from build123d import *

# Parameters (mm, degrees)
SKETCH1_R           = 7.67
BOSS_EXTRUDE1_DEPTH = 127
FILLET1_R           = 10
SKETCH2_W           = 50.8
SKETCH2_H           = 70.745219222
CUT_EXTRUDE1_DEPTH  = 186.59628229


with BuildPart() as part:
    # Sketch1 → Boss-Extrude1 (new body)
    with BuildSketch(Plane.XY):
        with BuildLine():
            Line((-19.5, 76.2), (-19.5, 0))
            ThreePointArc((-19.5, 0), (-13.788582233, -13.788582233), (0, -19.5))
            Line((0, -19.5), (76.2, -19.5))
            ThreePointArc((76.2, -19.5), (95.7, 0), (76.2, 19.5))
            Line((76.2, 19.5), (19.5, 19.5))
            Line((19.5, 19.5), (19.5, 76.2))
            ThreePointArc((19.5, 76.2), (0, 95.7), (-19.5, 76.2))
        make_face()
        Circle(SKETCH1_R, mode=Mode.SUBTRACT)
        with Locations((0, 76.2)):
            Circle(SKETCH1_R, mode=Mode.SUBTRACT)
        with Locations((76.2, 0)):
            Circle(SKETCH1_R, mode=Mode.SUBTRACT)
    extrude(amount=BOSS_EXTRUDE1_DEPTH)

    # Fillet1
    fillet1_edges = [part.edges().sort_by_distance(p)[0] for p in [
        (19.5, 19.5, 63.5),
    ]]
    fillet(fillet1_edges, radius=FILLET1_R)

    # Sketch2 → Cut-Extrude1 (cut, symmetric)
    with BuildSketch(Plane(origin=(0, 0, 0), x_dir=(0, 0, -1), z_dir=(1, 0, 0))):
        with Locations((-63.5, 80.272609611)):
            Rectangle(SKETCH2_W, SKETCH2_H)
    cut_extrude1 = extrude(amount=CUT_EXTRUDE1_DEPTH, both=True, mode=Mode.SUBTRACT)

    # Mirror1: Cut-Extrude1 across plane
    add(cut_extrude1.mirror(Plane(origin=(0, 0, 0), x_dir=(0, 0, 1), z_dir=(-0.7071067811865512, 0.7071067811865438, 0))), mode=Mode.SUBTRACT)


solid = part.part
Source: CAD feature listing. Evaluate the final solid. Frame: model axes, mm. A direction names the side the tool comes from. Coordinates: 2 decimals unless noted, no trailing zeros. Order: outer loops, then holes, each group sorted by start corner. A loop starts at its lowest first (then second) coordinate and runs counter-clockwise, first axis right, second up. Notation, with made-up numbers: M -37.75,-18 L 4.25,-18 A17 ccw 4.25,-6 Z; hole C 9.5,-7 d5. An arc over 180 degrees is marked long. Write each question's results on one line, items separated by ' | '. Start each with the question number.
Item 1: Line query: probe 1 along Y at (x, z) = (0, 24); probe 2 along Z at (x, y) = (16, 60); probe 3 along Y at (x, z) = (76.2, 117). Output: solid intervals per line, ascending.
Item 2: Cut plane D-D (y = 72). Return loops of the section in (x, z).
Item 3: Draft query along X for faces 1 (the face through (-13.939, -13.636, 62.611)), 2 (the face through (0, 64, 38.1)), 3 (the face through (-0.998, 83.805, 18.783)). Return one class per face: pulls with the +X half, pulls with the -X half, needs draft (parallel to the pull), parting line crosses it, or undercut.
Item 4: Cut plane B-B (y = 49.5). Return loops of the section in (x, z).
Item 5: Set-up query: faces 4 (the face through (24, 13, 127)), 5 (the face through (44.9, 0, 64)), 6 (the face through (0, 64, 88.9)). Return all of +Z, -Z, +X, -X, +Y, -Y with unobstructed straight access to the full face (end or side cutting, diameter ignored); none if empty.
Item 6: First-contact query: pin 1 Ø6 at (y, z) = (62.5, 105) entering from +X; pin 2 Ø1 at (x, z) = (32.5, 92.5) entering from +Y; pin 3 Ø12.5 at (x, y) = (0, 0) entering from -Z; pin 4 Ø8 at (x, z) = (84, 109) entering from +Y. Flat tips, straight axial feed; report the tip coordinate or a pass-through.
Item 7: Cut plane C-C (z = 68.5). Return loops of the section in (x, y).
Item 8: Cut plane A-A (z = 114.5). Return loops of the section in (x, y), and give its area (3 significant figures).
Checked values:
1) probe 1: y = -19.5 to -7.67, 7.67 to 68.53, 83.87 to 95.7 | probe 2: z = 0 to 38.1, 88.9 to 127 | probe 3: y = -19.5 to -7.67, 7.67 to 19.5
2) outline: M -19.5,0 L -6.42,0 L -6.42,38.1 L -19.5,38.1 Z; M -19.5,88.9 L -6.42,88.9 L -6.42,127 L -19.5,127 Z; M 6.42,0 L 19.5,0 L 19.5,38.1 L 6.42,38.1 Z; M 6.42,88.9 L 19.5,88.9 L 19.5,127 L 6.42,127 Z
3) face 1: pulls with the -X half | face 2: needs draft | face 3: undercut
4) outline: M -19.5,0 L 19.5,0 L 19.5,38.1 L -19.5,38.1 Z; M -19.5,88.9 L 19.5,88.9 L 19.5,127 L -19.5,127 Z
5) face 4: +Z, +X, -X, +Y, -Y | face 5: +X, +Y, -Y | face 6: +X, -X, +Y
6) pin 1: stops at x = 19.5 | pin 2: stops at y = 19.5 | pin 3: passes through | pin 4: stops at y = 19.13
7) outline: M -19.5,0 A19.5 ccw 0,-19.5 L 44.9,-19.5 L 44.9,19.5 L 29.5,19.5 A10 cw 19.5,29.5 L 19.5,44.9 L -19.5,44.9 Z; hole C 0,0 d15.34
8) outline: M -19.5,0 A19.5 ccw 0,-19.5 L 76.2,-19.5 A19.5 ccw 76.2,19.5 L 29.5,19.5 A10 cw 19.5,29.5 L 19.5,76.2 A19.5 ccw -19.5,76.2 Z; hole C 0,0 d15.34; hole C 0,76.2 d15.34; hole C 76.2,0 d15.34 | area: 6,520 mm2
